Work out the finished part from the listing and answer in its coordinate system (mm). A direction names the side the tool comes from. Give positions to 0.01 mm unless a question says otherwise; leave off trailing zeros. Write each loop counter-clockwise with the first axis right and the second up, starting at its lowest first coordinate (ties: lowest second). Pieces come first, ordered by that corner, then holes. Notation, with made-up numbers: (-34, 47.25) - (1, 47.25) arc R34 cw to (1, 82.25) - close; hole circle Ø7 at (63, -35.5). An arc over 180 degrees is marked (long way). Write item = value, one per line.
from build123d import *

# Parameters (mm, degrees)
CROQUIS1_W              = 67
CROQUIS1_H              = 51.82
SALIENTE_EXTRUIR1_DEPTH = 80
CORTAR_EXTRUIR1_REACH   = 69
CROQUIS4_W              = 60
CROQUIS4_H              = 30
CORTAR_EXTRUIR2_DEPTH   = 35
CORTAR_EXTRUIR3_REACH   = 69
CROQUIS5_W              = 45
CROQUIS5_H              = 5
CORTAR_EXTRUIR4_REACH   = 53.82
CORTAR_EXTRUIR5_REACH   = 53.82


with BuildPart() as part:
    # Croquis1 → Saliente-Extruir1 (new body)
    with BuildSketch(Plane(origin=(0, 0, 0), x_dir=(0, 0, -1), z_dir=(1, 0, 0))):
        with Locations((33.5, 25.91)):
            Rectangle(CROQUIS1_W, CROQUIS1_H)
    extrude(amount=SALIENTE_EXTRUIR1_DEPTH)

    # Croquis3 → Cortar-Extruir1 (cut, up to next)
    with BuildSketch(Plane.XY, mode=Mode.PRIVATE) as cortar_extruir1_sk1:
        Polygon((80, 0), (22.608406464, 30.515651581), (11.280683474, 51.82), (80, 51.82), align=None)
    cortar_extruir1_tool1 = extrude(cortar_extruir1_sk1.sketch, amount=-CORTAR_EXTRUIR1_REACH, mode=Mode.PRIVATE) & part.part
    add(cortar_extruir1_tool1.solids().sort_by_distance((53.313116, 33.143327, 0))[0], mode=Mode.SUBTRACT)

    # Croquis4 → Cortar-Extruir2 (cut)
    with BuildSketch(Plane(origin=(0, 51.82, 0), x_dir=(1, 0, 0), z_dir=(0, 1, 0))):
        with Locations((30, 33.5)):
            Rectangle(CROQUIS4_W, CROQUIS4_H)
    extrude(amount=-CORTAR_EXTRUIR2_DEPTH, mode=Mode.SUBTRACT)

    # Croquis5 → Cortar-Extruir3 (cut, up to next)
    with BuildSketch(Plane.XY, mode=Mode.PRIVATE) as cortar_extruir3_sk1:
        with Locations((22.5, 2.5)):
            Rectangle(CROQUIS5_W, CROQUIS5_H)
    cortar_extruir3_tool1 = extrude(cortar_extruir3_sk1.sketch, amount=-CORTAR_EXTRUIR3_REACH, mode=Mode.PRIVATE) & part.part
    add(cortar_extruir3_tool1.solids().sort_by_distance((22.5, 2.5, 0))[0], mode=Mode.SUBTRACT)

    # Croquis6 → Cortar-Extruir4 (cut, up to next)
    with BuildSketch(Plane(origin=(0, 51.82, 0), x_dir=(1, 0, 0), z_dir=(0, 1, 0)), mode=Mode.PRIVATE) as cortar_extruir4_sk1:
        Polygon((4.922856145, 67), (0, 64.334655313), (0, 67), align=None)
    cortar_extruir4_tool1 = extrude(cortar_extruir4_sk1.sketch, amount=-CORTAR_EXTRUIR4_REACH, mode=Mode.PRIVATE) & part.part
    add(cortar_extruir4_tool1.solids().sort_by_distance((1.640952, 51.82, -66.111552))[0], mode=Mode.SUBTRACT)

    # Croquis9 → Cortar-Extruir5 (cut, up to next)
    with BuildSketch(Plane(origin=(0, 51.82, 0), x_dir=(1, 0, 0), z_dir=(0, 1, 0)), mode=Mode.PRIVATE) as cortar_extruir5_sk1:
        Polygon((45, 67), (13.626202653, 52.370158031), (1.954435626, 52.832439456), (-4.658833913, 67.014641749), align=None)
    cortar_extruir5_tool1 = extrude(cortar_extruir5_sk1.sketch, amount=-CORTAR_EXTRUIR5_REACH, mode=Mode.PRIVATE) & part.part
    add(cortar_extruir5_tool1.solids().sort_by_distance((15.368059, 51.82, -61.265598))[0], mode=Mode.SUBTRACT)


solid = part.part
1. Find section B-B, the plane x = 9. Give the vertices of the cut face in (y, z).
Solution:
outline = (5, -52.55) - (51.82, -52.55) - (51.82, -48.5) - (16.82, -48.5) - (16.82, -18.5) - (51.82, -18.5) - (51.82, 0) - (5, 0) - close
2. Find section A-A, the plane z = -6. Give the vertices of the cut face in (x, y).
Solution:
outline = (0, 5) - (45, 5) - (45, 0) - (80, 0) - (22.61, 30.52) - (11.28, 51.82) - (0, 51.82) - close
3. Given pin 1 (5.5 mm diameter, centred on y = 2, z = -29, fed in from -X); pin 2 (22.5 mm diameter, centred on x = 28, z = -34.5, fed in from -Y); pin 3 (15 mm diameter, centred on x = 28, z = -37, fed in from +Y), each flat-ended and moving along its own axis, determine where each tip first touches the part or whether it passes through.
Solution:
pin_1 = 45
pin_2 = 5
pin_3 = 16.82
4. For a pull along Z with two mould halves and no side action, classify faces 1 (the flat face through (0.99, 28.74, -54.9)), 2 (the flat face through (13, 31, -48.5)), 3 (the flat face through (17.024, 41.019, -9.12)) as pulls with the +Z half, pulls with the -Z half, needs draft (parallel to the pull), parting line crosses it, or undercut.
Solution:
face_1 = pulls with the -Z half
face_2 = undercut
face_3 = needs draft
5. A tool of negligible diameter and unlimited length cuts with its end or side. For faces 4 (the flat face through (58, 7, -67)), 5 (the flat face through (13, 31, -18.5)), 6 (the flat face through (26.047, 17.077, -58.162)), 7 (the flat face through (45, 2, -33)), 8 (the flat face through (0, 24, -15)), from which of +Z, -Z, +X, -X, +Y, -Y can it reach the whole face along a straight path? Write none if from no direction.
Solution:
face_4 = -Z, +X, -X, +Y, -Y
face_5 = +X, -X, +Y
face_6 = -Z, +Y, -Y
face_7 = +Z, -Z, -X, -Y
face_8 = +Z, -Z, -X, +Y, -Y
6. Straight lines are drawn through the part: line 1 (Y direction, x = 10.5, z = -18); line 2 (Y direction, x = 36.5, z = -41); line 3 (Z direction, x = 11.5, y = 28.5). For each, find the intervals that lie inside material, in ascending order.
Solution:
line_1 = 5 to 51.82
line_2 = 5 to 16.82
line_3 = -52.45 to -48.5, -18.5 to 0
7. Find section C-C, the plane y = 12. Give the vertices of the cut face in (x, z).
Solution:
outline = (0, -57.02) - (1.95, -52.83) - (13.63, -52.37) - (45, -67) - (57.43, -67) - (57.43, 0) - (0, 0) - close
8. Find section D-D, the plane z = -46.5. Give the vertices of the cut face in (x, y), then the cut area to 3 significant figures.
Solution:
outline = (0, 5) - (45, 5) - (45, 0) - (80, 0) - (48.37, 16.82) - (0, 16.82) - close
area = 855 mm^2
